Check sheet for the drawn part. Datum: minimum x, y, z corner. Units: mm. A direction names the side the tool comes from. Coordinates: 2 decimals unless noted, no trailing zeros. Loops run counter-clockwise (first coordinate to the right, second up) from the corner with the lowest first, then second, coordinate; pieces in that order, holes last. Notation, with made-up numbers: (-10.75, 83.5) - (45.25, 83.5) arc R12 ccw to (45.25, 105.5) - close; hole circle Ø3 at (-39.5, 63). An arc over 180 degrees is marked (long way). Answer as CSV lines item,"result". Start each with the question number.
1. Cross-section at B-B (z = 8). Enter the section's corners in (x, y).
2. Material ranges on line 1 (Y direction, x = 19, z = 4); line 2 (X direction, y = 25.5, z = 12); line 3 (Z direction, x = 23.25, y = 18.5), recorded low to high. Write a range as [from, to].
3. Cross-section at C-C (y = 17). Enter the section's corners in (x, z).
4. Cross-section at A-A (y = 31.5). Enter the section's corners in (x, z), plus the area to 3 significant figures.
5. Set-up check for the marked faces 5, 6 and 7: record each of +Z, -Z, +X, -X, +Y, -Y from which the full face is reachable in a straight line by a thin tool's end or side.
6. Cross-section at D-D (x = 18.5). Enter the section's corners in (y, z).
7. Release check for a two-part mould opening along Z. For the marked faces 1, 2, 3 and 4 record: pulls with the +Z half, pulls with the -Z half, needs draft (parallel to the pull), parting line crosses it, or undercut.
8. Gauge pin test, flat ends, axial feed: P1, Ø10, axis at x = 8, y = 33, coming from the +Z side; P2, Ø10, axis at x = 10.5, y = 44.5, coming from the +Z side; P3, Ø2, axis at x = 7, y = 31.5, coming from the +Z side. Record the tip position at first contact, or that the pin passes through.
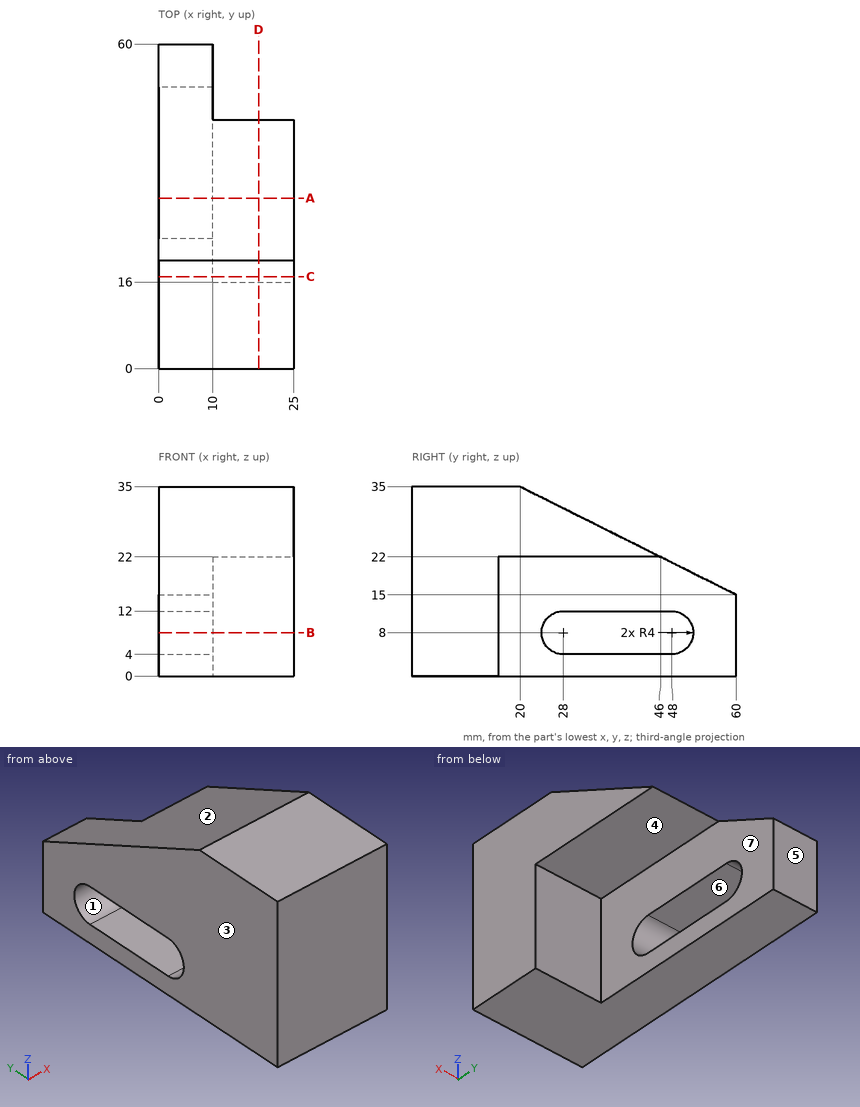
Values follow:
1,outline,"(0, 0) - (25, 0) - (25, 16) - (10, 16) - (10, 24) - (0, 24) - close; (0, 52) - (10, 52) - (10, 60) - (0, 60) - close"
2,line 1,"y = [0, 16]"
2,line 2,"x = [0, 10]"
2,line 3,"z = [22, 35]"
3,outline,"(0, 0) - (10, 0) - (10, 22) - (25, 22) - (25, 35) - (0, 35) - close"
4,outline,"(0, 0) - (10, 0) - (10, 4) - (0, 4) - close; (0, 12) - (10, 12) - (10, 22) - (25, 22) - (25, 29.25) - (0, 29.25) - close"
4,area,"321 mm²"
5,face 5,"+Z, -Z, +X, -X, +Y"
5,face 6,"+X, -X"
5,face 7,"-Z, +X, +Y"
6,outline,"(0, 0) - (16, 0) - (16, 22) - (46, 22) - (20, 35) - (0, 35) - close"
7,face 1,"undercut"
7,face 2,"pulls with the +Z half"
7,face 3,"needs draft"
7,face 4,"pulls with the -Z half"
8,P1,"stops at z = 31"
8,P2,"stops at z = 25.25"
8,P3,"stops at z = 29.75"
